Check sheet for the modelled part. Datum: model origin and axes. Units: mm. Face numbers are marked on the shaded views. Give positions to 0.01 mm unless a question says otherwise; leave off trailing zeros. Order: outer loops, then holes, each group sorted by start corner. A loop starts at its lowest first (then second) coordinate and runs counter-clockwise, first axis right, second up. Notation, with made-up numbers: (-5, -30.75) -> (24, -30.75) arc R34 cw to (24, 0.25) -> close; hole circle Ø7 at (4, 58). An arc over 180 degrees is marked (long way). One line per question, with ' | ' between items. Start each with the question number.
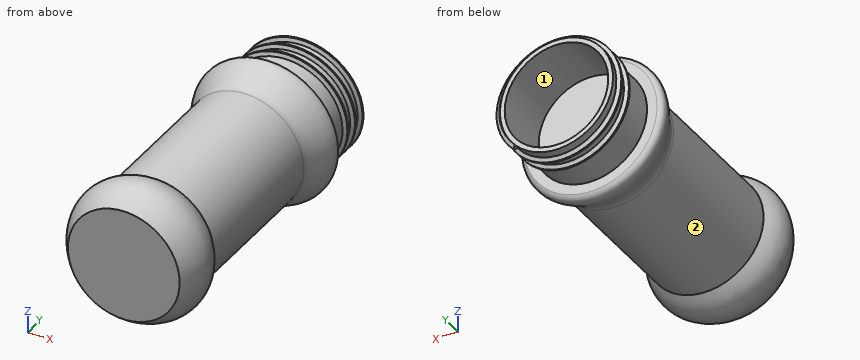
from build123d import *

# Parameters (mm, degrees)
SKETCH_3_R          = 17.85
EXTRUDE_1_DEPTH     = 47.5
SKETCH_5_R          = 17.2
SKETCH_5_R_2        = 15.75
EXTRUDE_2_DEPTH     = 18
SWEEP_6_PITCH       = 4
SWEEP_6_HEIGHT      = 10
SWEEP_6_RADIUS      = 17.2
SWEEP_6_START_ANGLE = 45


with BuildPart() as part:
    # По траектории5: sweep along a path in Эскиз1
    with BuildLine(Plane(origin=(0, 0, 0), x_dir=(1, 0, 0), z_dir=(0, 1, 0))) as sweep_5_path:
        CenterArc((0, 0), 20.25, 0, 360)
    # Эскиз2 → По траектории5 (sweep)
    with BuildSketch(Plane(origin=(0, 0, 20.25), x_dir=(0, 0, -1), z_dir=(1, 0, 0))):
        with BuildLine():
            Line((20.25, -2.884804654), (20.25, 13.715195346))
            Line((20.25, 13.715195346), (2.4, 13.715195346))
            add(Edge.make_bspline(
                [(3.25, -2.884804654), (-4.140339113, 5.721368346), (2.4, 13.715195346)],
                knots=[0, 0, 0, 1, 1, 1], degree=2))
            Line((3.25, -2.884804654), (20.25, -2.884804654))
        make_face()
    sweep(path=sweep_5_path.line)

    # Эскиз3 → Бобышка-Вытянуть1 (add)
    with BuildSketch(Plane(origin=(0, 13.715195346, 0), x_dir=(1, 0, 0), z_dir=(0, 1, 0))):
        Circle(SKETCH_3_R)
    extrude(amount=EXTRUDE_1_DEPTH)

    # Эскиз4 → Повернуть1 (revolve)
    with BuildSketch(Plane(origin=(0, 0, 20.25), x_dir=(0, 0, -1), z_dir=(1, 0, 0))):
        with BuildLine():
            add(Edge.make_bspline(
                [(2.4, 61.215195346), (3.008061282, 65.151641805), (-4.686382265, 72.118473987), (0, 74.215195346)],
                knots=[0, 0, 0, 0, 1, 1, 1, 1], degree=3))
            Line((0, 74.215195346), (20.25, 74.215195346))
            Line((20.25, 74.215195346), (20.25, 61.215195346))
            Line((20.25, 61.215195346), (2.4, 61.215195346))
        make_face()
    revolve(axis=Axis((0, 61.215195346, 0), (0, 1, 0)))

    # Эскиз5 → Бобышка-Вытянуть2 (add)
    with BuildSketch(Plane(origin=(0, 74.215195346, 0), x_dir=(1, 0, 0), z_dir=(0, 1, 0))):
        Circle(SKETCH_5_R)
        Circle(SKETCH_5_R_2, mode=Mode.SUBTRACT)
    extrude(amount=EXTRUDE_2_DEPTH)

    # По траектории6: sweep along a helix
    with BuildLine() as sweep_6_path:
        add(Helix(SWEEP_6_PITCH, SWEEP_6_HEIGHT, SWEEP_6_RADIUS, center=(0, 92.215195346, 0), direction=(0, -1, 0), mode=Mode.PRIVATE).rotate(Axis((0, 92.215195346, 0), (0, -1, 0)), SWEEP_6_START_ANGLE))
    # Эскиз9 → По траектории6 (sweep)
    with BuildSketch(Plane(origin=(12.162236636, 92.215195346, -12.162236636), x_dir=(0.705651254, -0.037044276, -0.707590298), z_dir=(0.706622929, -0.036987451, 0.706622929))):
        Polygon((0, 0.803706964), (0, -0.803706964), (1.2, -0.25), (1.2, 0.25), align=None)
    sweep(path=sweep_6_path.line, is_frenet=True)


solid = part.part
1. Go/stop test with flat-tipped pins: pin 1 (2 mm diameter, centred on y = 46.5, z = 14, fed in from +X); pin 2 (8 mm diameter, centred on y = 82, z = 10.5, fed in from -X) (3 decimals); pin 3 (1.5 mm diameter, centred on y = 83, z = 1, fed in from +X). Record where each tip stops, or that it passes through.
2. Cross-section at A-A on y = 77. Record the boundary of the cut face in (x, z), and give its area (3 significant figures).
3. Scan lines: probe 1 along Z at (x, y) = (0, 79); probe 2 along Y at (x, z) = (-4, 12.5). Record each from-to range of solid material in increasing order.
4. Mould release check, pull along X, two halves, no side actions. Record for the marked faces 1 and 2: +X half, -X half, draft (parallel to the pull), parting line (faces both ways), or undercut.
5. Cross-section at B-B on y = 28. Record the boundary of the cut face in (x, z), and give its area (3 significant figures).
Response values:
1) pin 1: stops at x = 12.23 | pin 2: stops at x = -15.975 | pin 3: stops at x = 18.39
2) outline: circle Ø34.4 at (0, 0); hole circle Ø31.5 at (0, 0) | area: 150 mm²
3) probe 1: z = -17.2 to -15.75, 15.75 to 17.2 | probe 2: y = -2.88 to 74.22
4) face 1: undercut | face 2: parting line
5) outline: circle Ø35.7 at (0, 0) | area: 1,000 mm²
